```python
from build123d import *

# Parameters (mm, degrees)
CROQUIS1_W                   = 40
CROQUIS1_H                   = 40
SALIENTE_EXTRUIR1_DEPTH      = 0.3
SALIENTE_EXTRUIR2_DEPTH      = 10
SALIENTE_EXTRUIR2_DEPTH_BACK = 10
CROQUIS2_R                   = 2.5
CORTAR_EXTRUIR1_DEPTH        = 2.5
CORTAR_EXTRUIR1_DEPTH_BACK   = 2.5
CROQUIS3_W                   = 14.056155144
CROQUIS3_H                   = 12
CROQUIS4_W                   = 300
CROQUIS4_H                   = 100
SALIENTE_EXTRUIR3_DEPTH      = 300
VACIADO2_START               = 4.3
VACIADO2_OUTLINE_W           = 292
VACIADO2_OUTLINE_H           = 96
VACIADO2_DEPTH               = 292
VACIADO2_START_2             = 4
VACIADO2_2_OUTLINE_W         = 32
VACIADO2_2_OUTLINE_H         = 32
VACIADO2_2_DEPTH             = 0.3
VACIADO2_3_OUTLINE_W         = 2
VACIADO2_3_OUTLINE_H         = 12
VACIADO2_3_DEPTH             = 4
CROQUIS6_W                   = 32
CROQUIS6_H                   = 32
SALIENTE_EXTRUIR4_DEPTH      = 0.3


with BuildPart() as part:
    # Croquis1 → Saliente-Extruir1 (new body)
    with BuildSketch(Plane.XY):
        Rectangle(CROQUIS1_W, CROQUIS1_H)
    extrude(amount=SALIENTE_EXTRUIR1_DEPTH)

    # Croquis2 → Saliente-Extruir2 (add, two sides: drawn at the far end of the back side and taken through both)
    with BuildSketch(Plane(origin=(0, 0, 0), x_dir=(1, 0, 0), z_dir=(0, 1, 0)).offset(-SALIENTE_EXTRUIR2_DEPTH_BACK)):
        with BuildLine():
            Line((-5, 10), (-5, 0))
            Line((-5, 0), (5, 0))
            Line((5, 0), (5, 10))
            ThreePointArc((5, 10), (0, 15), (-5, 10))
        make_face()
        with Locations(Location((0, 10, 0), (0, 0, 270))):
            Circle(CROQUIS2_R, mode=Mode.SUBTRACT)
    extrude(amount=SALIENTE_EXTRUIR2_DEPTH + SALIENTE_EXTRUIR2_DEPTH_BACK)

    # Croquis3 → Cortar-Extruir1 (cut, two sides: drawn at the far end of the back side and taken through both)
    with BuildSketch(Plane(origin=(0, 0, 0), x_dir=(1, 0, 0), z_dir=(0, 1, 0)).offset(-CORTAR_EXTRUIR1_DEPTH_BACK)):
        with Locations((0, 10)):
            Rectangle(CROQUIS3_W, CROQUIS3_H)
    extrude(amount=CORTAR_EXTRUIR1_DEPTH + CORTAR_EXTRUIR1_DEPTH_BACK, mode=Mode.SUBTRACT)

    # Croquis4 → Saliente-Extruir3 (add)
    with BuildSketch(Plane.XY.offset(0.3)):
        Rectangle(CROQUIS4_W, CROQUIS4_H)
    extrude(amount=SALIENTE_EXTRUIR3_DEPTH)

    # Vaciado2: read off the stored shape, not the designer's step
    # Vaciado2 outline → Vaciado2 (cut)
    with BuildSketch(Plane.XY.offset(VACIADO2_START)):
        with Locations((0, 2)):
            Rectangle(VACIADO2_OUTLINE_W, VACIADO2_OUTLINE_H)
    extrude(amount=VACIADO2_DEPTH, mode=Mode.SUBTRACT)

    # Vaciado2 2 outline → Vaciado2 2 (cut)
    with BuildSketch(Plane.XY.offset(VACIADO2_START_2)):
        Rectangle(VACIADO2_2_OUTLINE_W, VACIADO2_2_OUTLINE_H)
    extrude(amount=VACIADO2_2_DEPTH, mode=Mode.SUBTRACT)

    # Vaciado2 3 outline → Vaciado2 3 (cut)
    with BuildSketch(Plane.XY):
        Rectangle(VACIADO2_3_OUTLINE_W, VACIADO2_3_OUTLINE_H)
    extrude(amount=VACIADO2_3_DEPTH, mode=Mode.SUBTRACT)

    # Croquis6 → Saliente-Extruir4 (add)
    with BuildSketch(Plane.XY.offset(4)):
        Rectangle(CROQUIS6_W, CROQUIS6_H)
    extrude(amount=SALIENTE_EXTRUIR4_DEPTH)


solid = part.part
```
Source: CAD feature listing. Evaluate the final solid. Frame: model axes, mm. A direction names the side the tool comes from. Coordinates: 2 decimals unless noted, no trailing zeros. Order: outer loops, then holes, each group sorted by start corner. A loop starts at its lowest first (then second) coordinate and runs counter-clockwise, first axis right, second up. Notation, with made-up numbers: (-28.5, 65) - (8.5, 65) arc R30 ccw to (8.5, 100) - close; hole circle Ø9 at (81, 6). An arc over 180 degrees is marked (long way). One line per item, written item: value.
1) Cut plane D-D on y = -15. Output: boundary loops of the cut face in (x, z).
Computed values:
outline: (-150, 0.3) - (-20, 0.3) - (-20, 0) - (20, 0) - (20, 0.3) - (150, 0.3) - (150, 300.3) - (-150, 300.3) - close; hole (-146, 4.3) - (146, 4.3) - (146, 296.3) - (-146, 296.3) - close
2) Mould query, pull axis Z, two halves, no side actions, for faces 6 (the face through (0, -6, -15)), 7 (the face through (146, 1, 148)), 8 (the face through (0, -2.5, -7)). Classes: released by +Z, released by -Z, zero draft, split by the parting line, or undercut.
Computed values:
face 6: released by -Z
face 7: undercut
face 8: zero draft
3) Cut plane B-B on z = 52. Output: boundary loops of the cut face in (x, y).
Computed values:
outline: (-150, -50) - (150, -50) - (150, 50) - (146, 50) - (146, -46) - (-146, -46) - (-146, 50) - (-150, 50) - close
4) Cut plane C-C on x = -98. Output: boundary loops of the cut face in (y, z), plus the area to 3 significant figures.
Computed values:
outline: (-50, 0.3) - (50, 0.3) - (50, 4.3) - (-46, 4.3) - (-46, 296.3) - (50, 296.3) - (50, 300.3) - (-50, 300.3) - close
area: 1,970 mm^2
5) Cut plane A-A on y = -38. Output: boundary loops of the cut face in (x, z).
Computed values:
outline: (-150, 0.3) - (150, 0.3) - (150, 300.3) - (-150, 300.3) - close; hole (-146, 4.3) - (146, 4.3) - (146, 296.3) - (-146, 296.3) - close
6) Reachability of faces 1 (the face through (0, 2.5, -7)), 2 (the face through (5, -0.1, -3.8)), 3 (the face through (-2, 3, 296.3)), 4 (the face through (0, 10, -6)), 5 (the face through (-5, 0, -3)) from +Z, -Z, +X, -X, +Y, -Y: full face, straight path, thin tool, end or side. Return the list, or none.
Computed values:
face 1: -Z, +X, -X
face 2: -Z, +X, +Y, -Y
face 3: +Y
face 4: -Z, +X, -X, +Y
face 5: -Z, -X, +Y, -Y
7) Contact query for flat-ended pins moving along their axis: pin 1 (10 mm diameter, centred on x = 78, z = 268, fed in from +Y); pin 2 (5 mm diameter, centred on x = -0.5, z = -6.5, fed in from +Y); pin 3 (3 mm diameter, centred on x = 109, y = 35, fed in from -Z); pin 4 (11 mm diameter, centred on y = 4, z = -4.5, fed in from -X). Output: stop coordinate, or through.
Computed values:
pin 1: stops at y = -46
pin 2: stops at y = 10
pin 3: stops at z = 0.3
pin 4: stops at x = -150
8) Ray query, line 1 (Z direction, x = 0, y = -7); line 2 (X direction, y = 23.5, z = 283); line 3 (X direction, y = -8, z = -10). Return the intervals inside material, ascending. Write a range as [from, to].
Computed values:
line 1: z = [-15, -12.5], [-7.5, 4.3], [296.3, 300.3]
line 2: x = [-150, -146], [146, 150]
line 3: x = [-5, -2.5], [2.5, 5]
